Input: part model. Units: mm. Frame: model coordinates. A direction names the side the tool comes from. Coordinates: 2 decimals unless noted, no trailing zeros. Write each loop counter-clockwise with the first axis right and the second up, starting at its lowest first coordinate (ties: lowest second). Pieces come first, ordered by that corner, then holes.
from build123d import *

# Parameters (mm, degrees)
SKETCH2_R           = 330
SKETCH2_R_2         = 250
SKETCH2_W           = 44.45
SKETCH2_H           = 44.45
BOSS_EXTRUDE1_DEPTH = 10


with BuildPart() as part:
    # Sketch2 → Boss-Extrude1 (new body)
    with BuildSketch(Plane.XY):
        with Locations((-7.257473883, -45.051995239)):
            Circle(SKETCH2_R)
        with Locations((-7.257473883, -45.051995239)):
            Circle(SKETCH2_R_2, mode=Mode.SUBTRACT)
        Polygon((-272.796789122, 133.92041936), (-295.021789122, 95.425590162), (-256.526959924, 73.200590162), (-234.301959924, 111.69541936), align=None, mode=Mode.SUBTRACT)
        Polygon((258.281841356, 133.92041936), (219.787012158, 111.69541936), (242.012012158, 73.200590162), (280.506841356, 95.425590162), align=None, mode=Mode.SUBTRACT)
        with Locations((-7.257473883, -342.276995239)):
            Rectangle(SKETCH2_W, SKETCH2_H, mode=Mode.SUBTRACT)
    extrude(amount=BOSS_EXTRUDE1_DEPTH)


solid = part.part
Item 1: Section query B-B, the plane y = 187. Return loops of the section in (x, z).
Item 2: Pull-direction query (Y, two-part tool) for faces 1 (the face through (307.504, 54.071, 4.93)), 2 (the face through (-131, -264, 0)), 3 (the face through (269.55, 114.4, 4.93)); classes: released by +Y, released by -Y, zero draft, split by the parting line, or undercut.
Item 3: Section query D-D, the plane x = 1. Return loops of the section in (y, z).
Item 4: Access query for faces 4 (the face through (-245.57, 92.18, 4.93)), 5 (the face through (-131, -264, 10)). Directions: +Z, -Z, +X, -X, +Y, -Y. A direction counts if a zero-diameter tool reaches every point of the face in a straight line with its end or side. Return the directions, or none.
Item 5: Pin query (flat end, axial travel): pin 1 Ø6 at (x, z) = (-76, 4.5) entering from +Y; pin 2 Ø3 at (x, z) = (195.5, 4) entering from -Y; pin 3 Ø1.5 at (x, z) = (141, 5.5) entering from +Y; pin 4 Ø12 at (x, y) = (-226, -139.5) entering from -Z. Return the tip coordinate at first contact, or that it passes through.
Item 6: Section query A-A, the plane x = 127. Return loops of the section in (y, z), then the cut area to 3 significant figures.
Item 7: Material intervals for line 1 (Y direction, x = -11, z = 7.25); line 2 (X direction, y = 115, z = 4.25); line 3 (X direction, y = 152.5, z = 3), sorted ascending.
Item 8: Section query C-C, the plane z = 8.5. Return loops of the section in (x, y).
The answers:
1. outline: (-241.89, 0) - (-100.27, 0) - (-100.27, 10) - (-241.89, 10) - close; (85.76, 0) - (227.37, 0) - (227.37, 10) - (85.76, 10) - close
2. face 1: split by the parting line
2. face 2: zero draft
2. face 3: undercut
3. outline: (-374.95, 0) - (-364.5, 0) - (-364.5, 10) - (-374.95, 10) - close; (-320.05, 0) - (-294.92, 0) - (-294.92, 10) - (-320.05, 10) - close; (204.81, 0) - (284.84, 0) - (284.84, 10) - (204.81, 10) - close
4. face 4: +Z, -Z
4. face 5: +Z, +X, -X, +Y, -Y
5. pin 1: stops at y = 278.33
5. pin 2: stops at y = -306.58
5. pin 3: stops at y = 250.15
5. pin 4: passes through
6. outline: (-346.51, 0) - (-255.94, 0) - (-255.94, 10) - (-346.51, 10) - close; (165.84, 0) - (256.4, 0) - (256.4, 10) - (165.84, 10) - close
6. area: 1,810 mm2
7. line 1: y = -375.03 to -364.5, -320.05 to -295.02, 204.92 to 284.93
7. line 2: x = -295.85 to -283.72, -240.03 to -199.31, 184.79 to 225.51, 269.21 to 281.33
7. line 3: x = -271.59 to -160.47, 145.95 to 257.08
8. outline: circle Ø660 at (-7.26, -45.05); hole (-295.02, 95.43) - (-256.53, 73.2) - (-234.3, 111.7) - (-272.8, 133.92) - close; hole circle Ø500 at (-7.26, -45.05); hole (-29.48, -364.5) - (14.97, -364.5) - (14.97, -320.05) - (-29.48, -320.05) - close; hole (219.79, 111.7) - (242.01, 73.2) - (280.51, 95.43) - (258.28, 133.92) - close
